Can you work these out from the model? Positions are in its coordinate system, mm. Face numbers are marked on the shaded views. A direction names the side the tool comes from. Give positions to 0.01 mm unless a question says otherwise; leave off trailing zeros. Loops run counter-clockwise (first coordinate to the right, second up) from the corner with the lowest first, then second, coordinate; pieces in that order, holes last. Notation, with made-up numbers: (84, 66.25) - (130, 66.25) arc R17 cw to (130, 78.25) - close; hole circle Ø9 at (-31, 45.5). An arc over 180 degrees is marked (long way). Answer as a JSON object with one key per item and string values.
Autodesk Inventor part; units mm, degrees
ref_plane "YZ Plane" through (0, 0, 0) normal (1, 0, 0) x (0, 1, 0)
ref_plane "XZ Plane" through (0, 0, 0) normal (0, 1, 0) x (-1, 0, 0)
ref_plane "XY Plane" through (0, 0, 0) normal (0, 0, 1) x (1, 0, 0)
sketch "Sketch1" plane through (0, 0, 0) normal (0, 0, 1) x (1, 0, 0)
  circle A0 centre (0, 0) radius 26.5
  circle A1 centre (0, -150) radius 20
  line L0 (-26.4751, -1.1483) -> (-19.9812, -150.8667)
  line L1 (26.4751, -1.1483) -> (19.9812, -150.8667)
  line L2 (-15.5859, -21.432) -> (-10.7412, -133.1291)
  line L3 (15.5859, -21.432) -> (10.7412, -133.1291)
  line L4 (-5.5859, -25.9046) -> (14.5199, -46.0104)
  line L5 (-15.1953, -30.4373) -> (13.932, -59.5646)
  line L6 (-37.1, 0) -> (37.1, 0)
  line L7 (13.932, -59.5646) -> (-12.7736, -86.2702)
  line L8 (13.2907, -74.3479) -> (-12.1857, -99.8244)
  line L9 (-12.1857, -99.8244) -> (11.1726, -123.1827)
  line L10 (-11.5445, -114.6078) -> (4.3198, -130.4721)
  point P0 (-26.5, 0)
  point P1 (26.5, 0)
  dimension "d0" = 53
  dimension "d1" = 40
  dimension "d2" = 150
  dimension "d4" = 10
  dimension "d5" = 10
  dimension "d6" = 10
  dimension "d7" = 45
  dimension "d8" = 10
  dimension "d9" = 10
  dimension "d10" = 90
  dimension "d11" = 90
  dimension "d12" = 10
extrude "Extrusion1" add sketch "Sketch1" along normal blind 20 contours A0 L6 | A0 L2 A1 L0 | A0 L4 L3 L5 L2 | A0 L6 | A1 | A1 L3 A0 L1 | L7 L3 L8 L2 | L10 L2 L9 L3 A1
sketch "Sketch2" plane through (0, 0, 20) normal (0, 0, 1) x (1, 0, 0)
  line L0 (0, -209.3) -> (0, 65.8)
  line L1 (-6, 10.3923) -> (0, 0) construction
  point P0 (6, 10.3923)
  point P1 (-6, -10.3923)
  point P2 (-12, 0)
  point P3 (12, 0)
  point P4 (6, -10.3923)
  dimension "d18" = 12
  dimension "d19" = 12
  dimension "d22" = 360
hole "Hole1" at (-6, 10.3923, 20) at (-6, -10.3923, 20) at (-12, 0, 20) at (12, 0, 20) at (6, -10.3923, 20) at (6, 10.3923, 20) direction (0, 0, -1) diameter 4.5 end through all counterbore diameter 9.5 counterbore depth 5
fillet "Fillet1" radius 2 8 edges at (-15.1953, -30.4373, 10) (13.932, -59.5646, 10) (14.5199, -46.0104, 10) (-12.7736, -86.2702, 10) (13.2907, -74.3479, 10) (-12.1857, -99.8244, 10) (11.1726, -123.1827, 10) (-11.5445, -114.6078, 10)
chamfer "Chamfer3" distance 1 angle 45 6 edges at (-12, 4.75, 20) (-6, -5.6423, 20) (-6, 15.1423, 20) (6, -5.6423, 20) (6, 15.1423, 20) (12, 4.75, 20)
chamfer "Chamfer2" distance 5 angle 45 4 edges at (23.2282, -76.0075, 20) (0, 26.5, 20) (-23.2282, -76.0075, 20) (0, -170, 20)
sketch "Sketch3" plane through (0, 0, 20) normal (0, 0, 1) x (1, 0, 0)
  arc A0 (-14.9859, -150.65) -> (14.9859, -150.65) centre (0, -150) ccw
  point P0 (0, 0)
hole "Hole2" at (0, -150, 20) direction (0, 0, -1) diameter 10 end through all counterbore diameter 22 counterbore depth 8
chamfer "Chamfer4" distance 1.5 angle 45 1 edges at (0, -139, 20)
properties part number "UPPER_LINKAGE_LH"
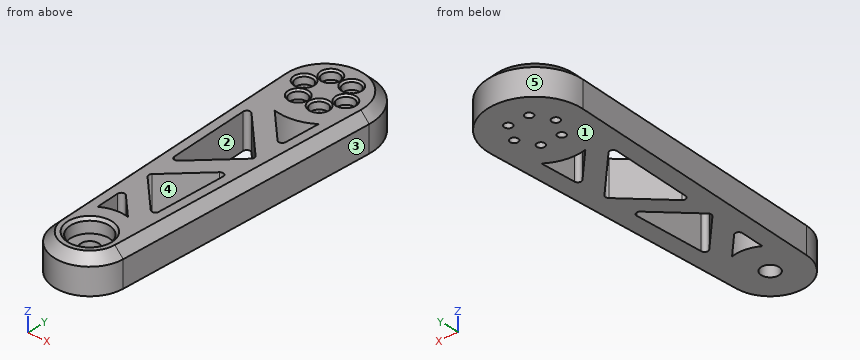
1) Imagine slicing it at B-B on z = 2.25. Give the number of separate pieces and of enclosed holes in the cut face, and give its area (3 significant figures).
Check sheet entries:
{"separate pieces": "1", "enclosed holes": "11", "area": "6,850 mm2"}
2) I need wall thicknesses on L1, parallel to X at y = 0, z = 11.25; L2, parallel to Y at x = -12, z = 11; L3, parallel to X at y = -82, z = 19.25. Which ranges of each line are inside material? Lowest first, please.
Check sheet entries:
{"L1": "-26.5 to -14.25, -9.75 to 9.75, 14.25 to 26.5", "L2": "-166 to -83.36, -33.74 to -2.25, 2.25 to 23.63", "L3": "-18.71 to -12.94, -8.5 to 5.64, 12.96 to 18.71"}
3) Imagine slicing it at A-A on y = -48. Write out the boundary of the cut face in (x, z).
Check sheet entries:
{"outline": "(-24.44, 0) - (-14.43, 0) - (-14.43, 20) - (-19.44, 20) - (-24.44, 15) - close; (2.37, 0) - (24.44, 0) - (24.44, 15) - (19.44, 20) - (2.37, 20) - close"}
4) If we mould it in two halves opening along X, with no side actions, what happens to the marked faces 3, 4 and 5? For each: released by +X, released by -X, zero draft, split by the parting line, or undercut.
Check sheet entries:
{"face 3": "released by +X", "face 4": "undercut", "face 5": "split by the parting line"}
5) I'm going to push flat-ended pins straight in: P1, Ø6, axis at y = -83, z = 9, coming from the +X side (3 decimals); P2, Ø7.5, axis at x = 12, y = 0, coming from the -Z side; P3, Ø10, axis at y = -24.5, z = 10, coming from the +X side; P4, Ø6, axis at x = -4, z = 12, coming from the +Y side. Where does each tip first touch, or does it pass through?
Check sheet entries:
{"P1": "x = 23.055", "P2": "z = 0", "P3": "x = 25.68", "P4": "y = 26.48"}
6) Which directions (+Z, -Z, +X, -X, +Y, -Y) give clear straight access to the entire face, cutting with the end or side of a thin tool? Please do the marked faces 1 and 2.
Check sheet entries:
{"face 1": "-Z, +X, -X, +Y, -Y", "face 2": "+Z, -Z"}
